```python
from build123d import *

# Parameters (mm, degrees)
SKETCH_1_R          = 5.85
EXTRUDE_1_DEPTH     = 1.4
SKETCH_2_R          = 4.6
EXTRUDE_2_DEPTH     = 2
SKETCH_3_R          = 4.9
EXTRUDE_3_DEPTH     = 5.9
SKETCH_4_R          = 10.526345736
SKETCH_4_R_2        = 4.5
CUT_EXTRUDE_1_DEPTH = 1
CUT_EXTRUDE_2_DEPTH = 2
SKETCH_6_R          = 3
EXTRUDE_4_DEPTH     = 5


with BuildPart() as part:
    # 草图1 → 凸台-拉伸1 (new body)
    with BuildSketch(Plane(origin=(0, 0, 0), x_dir=(1, 0, 0), z_dir=(0, 1, 0))):
        Circle(SKETCH_1_R)
    extrude(amount=EXTRUDE_1_DEPTH)

    # 草图2 → 凸台-拉伸2 (add)
    with BuildSketch(Plane(origin=(0, 1.4, 0), x_dir=(1, 0, 0), z_dir=(0, 1, 0))):
        Circle(SKETCH_2_R)
    extrude(amount=EXTRUDE_2_DEPTH)

    # 草图3 → 凸台-拉伸3 (add)
    with BuildSketch(Plane(origin=(0, 3.4, 0), x_dir=(1, 0, 0), z_dir=(0, 1, 0))):
        Circle(SKETCH_3_R)
    extrude(amount=EXTRUDE_3_DEPTH)

    # 草图4 → 切除-拉伸1 (cut)
    with BuildSketch(Plane.XZ.offset(-3.4)):
        Circle(SKETCH_4_R)
        Circle(SKETCH_4_R_2, mode=Mode.SUBTRACT)
    extrude(amount=-CUT_EXTRUDE_1_DEPTH, mode=Mode.SUBTRACT)

    # 草图5 → 切除-拉伸2 (cut)
    with BuildSketch(Plane(origin=(0, 9.3, 0), x_dir=(1, 0, 0), z_dir=(0, 1, 0))):
        Polygon((-3.702575932, 0), (-1.851287966, -3.206524817), (1.851287966, -3.206524817), (3.702575932, 0), (1.851287966, 3.206524817), (-1.851287966, 3.206524817), align=None)
    extrude(amount=-CUT_EXTRUDE_2_DEPTH, mode=Mode.SUBTRACT)

    # 草图6 → 凸台-拉伸4 (add)
    with BuildSketch(Plane.XZ):
        Circle(SKETCH_6_R)
    extrude(amount=EXTRUDE_4_DEPTH)


solid = part.part
```
The listing builds one solid part. Answer for the finished solid, in the listing's coordinates (mm). A direction names the side the tool comes from. Round coordinates to 2 decimals unless told otherwise and drop trailing zeros. Order: outer loops, then holes, each group sorted by start corner. A loop starts at its lowest first (then second) coordinate and runs counter-clockwise, first axis right, second up. Notation, with made-up numbers: (7, -24) - (46, -24) arc R19 cw to (46, -14) - close; hole circle Ø9 at (78, -14). An arc over 180 degrees is marked (long way). Put each result on its own line as item: value. Start each with the question number.
(1) Find section B-B (z = 3.5). Give the vertices of the cut face in (x, y).
(2) For faces 1 (the flat face through (0, -5, 0)), 2 (the cylindrical face through (-1.27, 0.69, 5.71)), 3 (the flat face through (3, 1.4, 4)), 4 (the cylindrical face through (-3, -2, 0)), 5 (the flat face through (2.79, 8.31, -1.58)), determine the directions among +Z, -Z, +X, -X, +Y, -Y from which every point of the face is accessible in a straight line to the end or side of a thin tool.
(3) Straight lines are drawn through the part: probe 1 along Y at (x, z) = (3.75, 2); probe 2 along Y at (x, z) = (-1, 5.5); probe 3 along X at (y, z) = (8.5, 3.5). For each, find the intervals that lie inside material, in ascending order. Write a range as from..to.
(4) Find section C-C (y = 0.25). Give the vertices of the cut face in (x, z).
(5) Find section A-A (x = 0). Give the vertices of the cut face in (y, z).
(6) Find section D-D (x = 3.25). Give the vertices of the cut face in (y, z), plus the area to 3 significant figures.
(7) Determine the mould class of faces 6 (the flat face through (-3, 0, -1)), 7 (the cylindrical face through (-1.062, 6.816, 4.783)), 8 (the flat face through (0, 8, 3.207)) for opening direction X: released by +X, released by -X, zero draft, split by the parting line, or undercut.
(8) Given P1, Ø0.6, axis at x = 0.5, y = 8.5, coming from the -Z side; P2, Ø4, axis at x = 2.5, y = 3, coming from the +Z side; P3, Ø5, axis at x = 4.5, y = 0.5, coming from the -Z side, each flat-ended and moving along its own axis, determine where each tip first touches the part or whether it passes through.
Reply:
1. outline: (-4.69, 0) - (4.69, 0) - (4.69, 1.4) - (2.98, 1.4) - (2.98, 3.4) - (2.83, 3.4) - (2.83, 4.4) - (3.43, 4.4) - (3.43, 9.3) - (-3.43, 9.3) - (-3.43, 4.4) - (-2.83, 4.4) - (-2.83, 3.4) - (-2.98, 3.4) - (-2.98, 1.4) - (-4.69, 1.4) - close
2. face 1: +Z, -Z, +X, -X, -Y
2. face 2: +Y, -Y
2. face 3: none
2. face 4: -Y
2. face 5: +Y
3. probe 1: 0..9.3
3. probe 2: 0..1.4
3. probe 3: -3.43..3.43
4. outline: circle Ø11.7 at (0, 0)
5. outline: (-5, -3) - (0, -3) - (0, -5.85) - (1.4, -5.85) - (1.4, -4.6) - (3.4, -4.6) - (3.4, -4.5) - (4.4, -4.5) - (4.4, -4.9) - (9.3, -4.9) - (9.3, -3.21) - (7.3, -3.21) - (7.3, 3.21) - (9.3, 3.21) - (9.3, 4.9) - (4.4, 4.9) - (4.4, 4.5) - (3.4, 4.5) - (3.4, 4.6) - (1.4, 4.6) - (1.4, 5.85) - (0, 5.85) - (0, 3) - (-5, 3) - close
6. outline: (0, -4.86) - (1.4, -4.86) - (1.4, -3.26) - (3.4, -3.26) - (3.4, -3.11) - (4.4, -3.11) - (4.4, -3.67) - (9.3, -3.67) - (9.3, -0.78) - (7.3, -0.78) - (7.3, 0.78) - (9.3, 0.78) - (9.3, 3.67) - (4.4, 3.67) - (4.4, 3.11) - (3.4, 3.11) - (3.4, 3.26) - (1.4, 3.26) - (1.4, 4.86) - (0, 4.86) - close
6. area: 65.7 mm^2
7. face 6: zero draft
7. face 7: split by the parting line
7. face 8: undercut
8. P1: z = -4.9
8. P2: z = 5.7
8. P3: z = -5.5
